Could you check a few things on this model? Use its own coordinates, in mm. Face numbers are marked on the shaded views. A direction names the side the tool comes from. Give positions to 0.01 mm unless a question says otherwise; leave off trailing zeros. Write each loop counter-clockwise with the first axis right and the second up, starting at its lowest first coordinate (ties: lowest second). Pieces come first, ordered by that corner, then holes. Notation, with made-up numbers: M 56.5,72.25 L 85.5,72.25 A25 cw 85.5,99.25 Z; hole C 5.25,7 d7. An arc over 180 degrees is marked long. Use one line per item in the form item = value.
from build123d import *

# Parameters (mm, degrees)
SKETCH_4_OUTSIDE_W   = 65.512
SKETCH_4_OUTSIDE_H   = 65.512
SKETCH_4_OUTSIDE_W_2 = 6
SKETCH_4_OUTSIDE_H_2 = 5.5
CUT_EXTRUDE_2_DEPTH  = 12
SKETCH_5_R           = 1.5
CUT_EXTRUDE_3_DEPTH  = 5


with BuildPart() as part:
    # Эскиз1 → Повернуть1 (revolve)
    with BuildSketch(Plane.XY, mode=Mode.PRIVATE) as revolve_1_sk:
        Polygon((0, 0), (-9, 0), (-9, -1.5), (-18, -1.5), (-18, -21.5), (-18.5, -21.5), (-18.5, -56.5), (-18, -56.5), (-18, -58.5), (-16, -58.5), (-16, -62.8), (-17.5, -62.8), (-17.5, -100.8), (-16, -100.8), (-16, -104.8), (-10, -104.8), (-10, -106.8), (-3, -106.8), (-3, -121.8), (0, -121.8), align=None)
    revolve(revolve_1_sk.sketch.rotate(Axis((0, -180.909291234, 0), (0, 1, 0)), 270), axis=Axis((0, -180.909291234, 0), (0, 1, 0)))

    # Эскиз4 outside → Вырез-Вытянуть2 (cut)
    with BuildSketch(Plane.XZ.offset(121.8)):
        Rectangle(SKETCH_4_OUTSIDE_W, SKETCH_4_OUTSIDE_H)
        Rectangle(SKETCH_4_OUTSIDE_W_2, SKETCH_4_OUTSIDE_H_2, mode=Mode.SUBTRACT)
    extrude(amount=-CUT_EXTRUDE_2_DEPTH, mode=Mode.SUBTRACT)

    # Эскиз5 → Вырез-Вытянуть3 (cut)
    with BuildSketch(Plane.XZ.offset(104.8)):
        with Locations(Location((-9, 9, 0), (0, 0, 270))):
            Circle(SKETCH_5_R)
        with Locations(Location((9, 9, 0), (0, 0, 270))):
            Circle(SKETCH_5_R)
        with Locations(Location((9, -9, 0), (0, 0, 270))):
            Circle(SKETCH_5_R)
        with Locations(Location((-9, -9, 0), (0, 0, 270))):
            Circle(SKETCH_5_R)
    extrude(amount=-CUT_EXTRUDE_3_DEPTH, mode=Mode.SUBTRACT)


solid = part.part
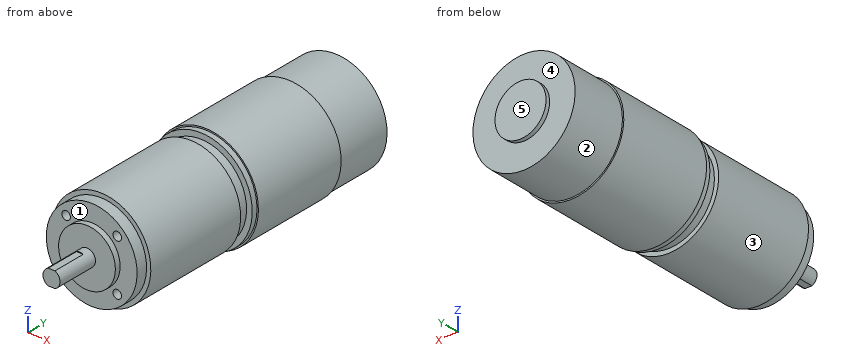
1) If I drill on L1, parallel to X at y = -103.75, z = -9; L2, parallel to Y at x = -6, z = 15; L3, parallel to X at y = -61.5, z = 12.5, over which ranges is the centre line in solid material (lowest first)?
Checked values:
L1 = -13.23 to -10.5, -7.5 to 7.5, 10.5 to 13.23
L2 = -100.8 to -62.8, -58.5 to -1.5
L3 = -9.99 to 9.99
2) I want a section at A-A, the plane x = 12. Please give me the cut outline in (y, z), plus the area to 3 significant figures.
Checked values:
outline = M -104.8,-10.58 L -100.8,-10.58 L -100.8,-12.74 L -62.8,-12.74 L -62.8,-10.58 L -58.5,-10.58 L -58.5,-13.42 L -56.5,-13.42 L -56.5,-14.08 L -21.5,-14.08 L -21.5,-13.42 L -1.5,-13.42 L -1.5,13.42 L -21.5,13.42 L -21.5,14.08 L -56.5,14.08 L -56.5,13.42 L -58.5,13.42 L -58.5,10.58 L -62.8,10.58 L -62.8,12.74 L -100.8,12.74 L -100.8,10.58 L -104.8,10.58 Z
area = 2,720 mm2
3) Thinking about a two-plate mould opening in Z: for the marked faces 1 and 2, which applies, released by +Z, released by -Z, zero draft, split by the parting line, or undercut?
Checked values:
face_1 = zero draft
face_2 = split by the parting line
4) For pin 1 Ø3 at (y, z) = (-103, -3.5) entering from +X; pin 2 Ø4 at (x, y) = (4, -29) entering from +Z; pin 3 Ø2.5 at (x, z) = (-9.5, -9.5) entering from -Y, each with a flat end and sliding along its axis, tell me the tip position at first contact or that it passes through.
Checked values:
pin_1 = 15.87
pin_2 = 18.39
pin_3 = -104.8
5) I want a section at B-B, the plane y = -91.5. Please give me the cut outline in (x, z).
Checked values:
outline = C 0,0 d35
6) For the marked faces 3, 4 and 5, which set-ups out of +Z, -Z, +X, -X, +Y, -Y let a thin tool reach every point of the face, with its end or its side?
Checked values:
face_3 = -Y
face_4 = +Y
face_5 = +Z, -Z, +X, -X, +Y
